Check sheet for the modelled part. Datum: model origin and axes. Units: mm. Face numbers are marked on the shaded views. A direction names the side the tool comes from. Give positions to 0.01 mm unless a question says otherwise; leave off trailing zeros. Loops run counter-clockwise (first coordinate to the right, second up) from the corner with the lowest first, then second, coordinate; pieces in that order, holes last. Notation, with made-up numbers: (-10.5, 26.5) - (5.5, 26.5) arc R20 ccw to (5.5, 57.5) - close; hole circle Ø11 at (-8, -1.5). An arc over 180 degrees is marked (long way). Use CSV: the item, a comma, the result in double quotes.
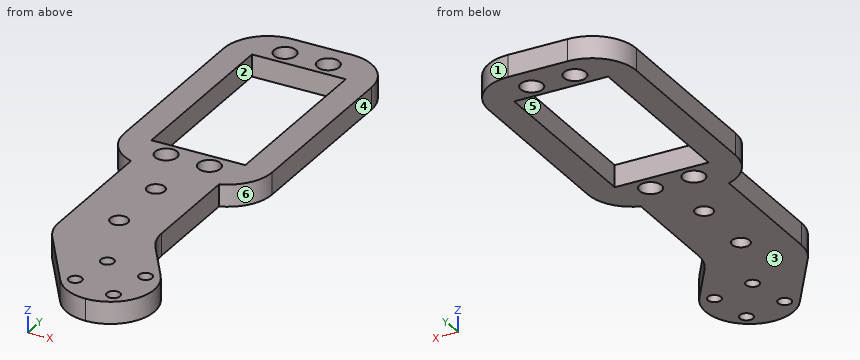
from build123d import *

# Parameters (mm, degrees)
BOSS_EXTRUDE1_DEPTH = 5
SKETCH4_W           = 33.55861501
SKETCH4_H           = 60
BOSS_EXTRUDE2_DEPTH = 5
SKETCH3_R           = 2.5
SKETCH3_W           = 21.3
SKETCH3_H           = 41
CUT_EXTRUDE1_DEPTH  = 5
FILLET1_R           = 10
SKETCH2_R           = 1.5
SKETCH2_R_2         = 2
CUT_EXTRUDE2_DEPTH  = 5
FILLET2_R           = 10


with BuildPart() as part:
    # Sketch1 → Boss-Extrude1 (new body)
    with BuildSketch(Plane.XY):
        with BuildLine():
            Line((-20.15, 104.620325978), (-20.15, 11.934589711))
            Line((-20.15, 11.934589711), (-8.282080395, -5.604207734))
            ThreePointArc((-8.282080395, -5.604207734), (-4.754289632, -8.797541139), (-0.15, -9.998874937))
            ThreePointArc((-0.15, -9.998874937), (8.797541139, -4.754289632), (8.282080395, 5.604207734))
            Line((8.282080395, 5.604207734), (-0.15, 18.065410289))
            Line((-0.15, 18.065410289), (-0.15, 104.620325978))
            Line((-0.15, 104.620325978), (-20.15, 104.620325978))
        make_face()
    extrude(amount=BOSS_EXTRUDE1_DEPTH)

    # Sketch4 → Boss-Extrude2 (add)
    with BuildSketch(Plane.XY.offset(5)):
        with Locations((-10.15, 74.620325978)):
            Rectangle(SKETCH4_W, SKETCH4_H)
    extrude(amount=-BOSS_EXTRUDE2_DEPTH)

    # Sketch3 → Cut-Extrude1 (cut)
    with BuildSketch(Plane.XY.offset(5)):
        with Locations((-5.55, 50.370325978)):
            Circle(SKETCH3_R)
        with Locations((-15.37372371, 50.370325978)):
            Circle(SKETCH3_R)
        with Locations((-15.37372371, 98.870325978)):
            Circle(SKETCH3_R)
        with Locations((-5.55, 98.870325978)):
            Circle(SKETCH3_R)
        with Locations((-10.15, 74.620325978)):
            Rectangle(SKETCH3_W, SKETCH3_H)
    extrude(amount=-CUT_EXTRUDE1_DEPTH, mode=Mode.SUBTRACT)

    # Fillet1
    # the kernel refuses this fillet: 10 mm, written as the material it takes off along each edge
    with BuildSketch(Plane(origin=(-26.929307505, 104.620325978, 30), x_dir=(1, 0, 0), z_dir=(0, 0, -1))) as fillet1_piece_1:
        with BuildLine():
            CenterArc((FILLET1_R, FILLET1_R), FILLET1_R, 180, 90)
            Line((0, FILLET1_R), (-FILLET1_R * 0.02, FILLET1_R))
            Line((-FILLET1_R * 0.02, FILLET1_R), (-FILLET1_R * 0.02, -FILLET1_R * 0.02))
            Line((-FILLET1_R * 0.02, -FILLET1_R * 0.02), (FILLET1_R, -FILLET1_R * 0.02))
            Line((FILLET1_R, -FILLET1_R * 0.02), (FILLET1_R, 0))
        make_face()
    extrude(amount=55, mode=Mode.SUBTRACT)
    with BuildSketch(Plane(origin=(6.629307505, 104.620325978, 30), x_dir=(-1, 0, 0), z_dir=(0, 0, -1))) as fillet1_piece_2:
        with BuildLine():
            CenterArc((FILLET1_R, -FILLET1_R), FILLET1_R, 90, 90)
            Line((0, -FILLET1_R), (-FILLET1_R * 0.02, -FILLET1_R))
            Line((-FILLET1_R * 0.02, -FILLET1_R), (-FILLET1_R * 0.02, FILLET1_R * 0.02))
            Line((-FILLET1_R * 0.02, FILLET1_R * 0.02), (FILLET1_R, FILLET1_R * 0.02))
            Line((FILLET1_R, FILLET1_R * 0.02), (FILLET1_R, 0))
        make_face()
    extrude(amount=55, mode=Mode.SUBTRACT)
    with BuildSketch(Plane(origin=(6.629307505, 44.620325978, 28.667902824), x_dir=(0, 1, 0), z_dir=(0, 0, -1))) as fillet1_piece_3:
        with BuildLine():
            CenterArc((9.46716113, -10), FILLET1_R, 90, 71.211889426)
            Line((0, -6.779307505), (-0.189343223, -6.714893655))
            ThreePointArc((-0.189343223, -6.714893655), (-0.2, -3.389653753), (-0.2, 0))
            Line((-0.2, 0), (0, 0.2))
            Line((0, 0.2), (9.46716113, 0.2))
            Line((9.46716113, 0.2), (9.46716113, 0))
        make_face()
    extrude(amount=52.335805648, mode=Mode.SUBTRACT)
    with BuildSketch(Plane(origin=(-26.929307505, 44.620325978, 28.667902824), x_dir=(0, 1, 0), z_dir=(0, 0, -1))) as fillet1_piece_4:
        with BuildLine():
            CenterArc((9.46716113, 10), FILLET1_R, 198.788110574, 71.211889426)
            Line((0, 6.779307505), (-0.189343223, 6.714893655))
            ThreePointArc((-0.189343223, 6.714893655), (-0.2, 3.389653753), (-0.2, 0))
            Line((-0.2, 0), (0, -0.2))
            Line((0, -0.2), (9.46716113, -0.2))
            Line((9.46716113, -0.2), (9.46716113, 0))
        make_face()
    extrude(amount=52.335805648, mode=Mode.SUBTRACT)

    # Sketch2 → Cut-Extrude2 (cut)
    with BuildSketch(Plane.XY.offset(5)):
        with Locations((-3.922945414, 5.797456277)):
            Circle(SKETCH2_R)
        with Locations((5.797456277, 3.922945414)):
            Circle(SKETCH2_R)
        with Locations((3.922945414, -5.797456277)):
            Circle(SKETCH2_R)
        with Locations((-5.797456277, -3.922945414)):
            Circle(SKETCH2_R)
        with Locations((-10.15, 21.797456277)):
            Circle(SKETCH2_R_2)
        with Locations((-10.15, 36.797456277)):
            Circle(SKETCH2_R_2)
    extrude(amount=-CUT_EXTRUDE2_DEPTH, mode=Mode.SUBTRACT)

    # Fillet2
    fillet2_edges = [part.edges().sort_by_distance(p)[0] for p in [
        (-20.15, 11.934589711, 2.5),
        (-0.15, 18.065410289, 2.5),
    ]]
    fillet(fillet2_edges, radius=FILLET2_R)


solid = part.part
1. Release check for a two-part mould opening along Y. For the marked faces 1, 2 and 3 record: released by +Y, released by -Y, zero draft, split by the parting line, or undercut.
Completed:
face 1,"released by +Y"
face 2,"undercut"
face 3,"zero draft"
2. Set-up check for the marked faces 4, 5 and 6: record each of +Z, -Z, +X, -X, +Y, -Y from which the full face is reachable in a straight line by a thin tool's end or side.
Completed:
face 4,"+Z, -Z, +X, +Y"
face 5,"+Z, -Z"
face 6,"+Z, -Z, +X"
3. Go/stop test with flat-tipped pins: pin 1 Ø2.5 at (y, z) = (30.5, 2.5) entering from +X; pin 2 Ø2 at (x, z) = (-21, 0.5) entering from +Y; pin 3 Ø1.5 at (y, z) = (1.5, 1) entering from -X. Record where each tip stops, or that it passes through.
Completed:
pin 1,"stops at x = -0.15"
pin 2,"stops at y = 104.14"
pin 3,"stops at x = -13.6"
4. Sectioned sample at D-D, the plane x = -22.5. Record the boundary of the cut face in (y, z), and give its area (3 significant figures).
Completed:
outline,"(45.78, 0) - (102.92, 0) - (102.92, 5) - (45.78, 5) - close"
area,"286 mm²"
5. Sectioned sample at A-A, the plane y = 87.5. Record the boundary of the cut face in (x, z).
Completed:
outline,"(-26.93, 0) - (-20.8, 0) - (-20.8, 5) - (-26.93, 5) - close; (0.5, 0) - (6.63, 0) - (6.63, 5) - (0.5, 5) - close"
6. Sectioned sample at C-C, the plane x = -10.15. Record the boundary of the cut face in (y, z), and give its area (3 significant figures).
Completed:
outline,"(-2.84, 0) - (19.8, 0) - (19.8, 5) - (-2.84, 5) - close; (23.8, 0) - (34.8, 0) - (34.8, 5) - (23.8, 5) - close; (38.8, 0) - (54.12, 0) - (54.12, 5) - (38.8, 5) - close; (95.12, 0) - (104.62, 0) - (104.62, 5) - (95.12, 5) - close"
area,"292 mm²"
7. Scan lines: line 1 along Y through (x, z) = (-7.5, 2.3); line 2 along Y through (x, z) = (-6.5, 3.1); line 3 along X through (y, z) = (75.5, 4). Record each from-to range of solid material in increasing order.
Completed:
line 1,"y = -6.61 to 48.81, 51.93 to 54.12, 95.12 to 97.31, 100.43 to 104.62"
line 2,"y = -7.6 to -5.25, -2.6 to 48.06, 52.68 to 54.12, 95.12 to 96.56, 101.18 to 104.62"
line 3,"x = -26.93 to -20.8, 0.5 to 6.63"
8. Sectioned sample at B-B, the plane z = 3.9. State how many separate pieces and enclosed holes the cut face has, and give its area (3 significant figures).
Completed:
separate pieces,"1"
enclosed holes,"11"
area,"2,040 mm²"
